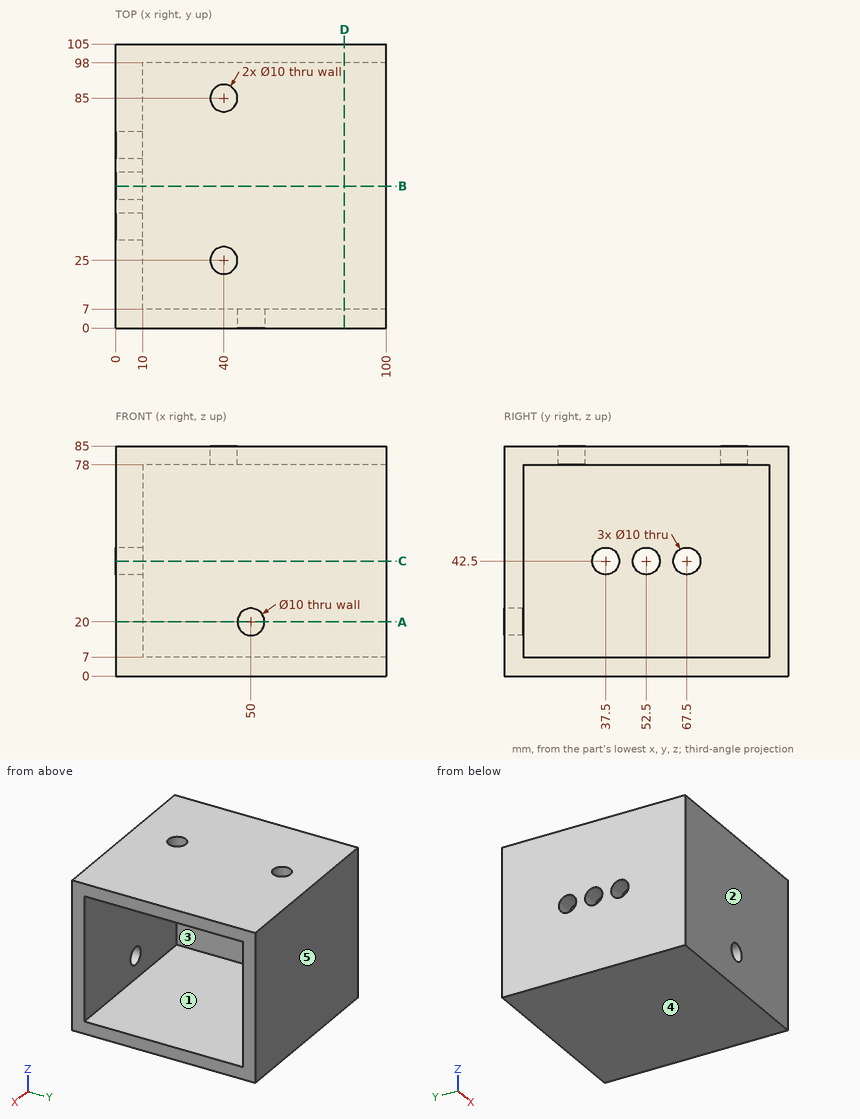
The figure shows three views and two pictorial views of one solid part (mm, origin at its lowest corner). Answer the questions. A direction names the side the tool comes from. Round coordinates to 2 decimals unless told otherwise and drop trailing zeros. Write each loop counter-clockwise with the first axis right and the second up, starting at its lowest first coordinate (ties: lowest second). Pieces come first, ordered by that corner, then holes. Notation, with made-up numbers: (30.25, -19.5) - (62.25, -19.5) arc R16 ccw to (62.25, 2.5) - close; hole circle Ø6 at (31, 55). An arc over 180 degrees is marked (long way). Use one line per item in the form item = value. Start each with the question number.
Item 1: A cutting plane is placed at A-A (z = 20). Write down the section's boundary in (x, y).
Item 2: Determine the mould class of the marked faces 3, 4 and 5 for opening direction Y: +Y half, -Y half, draft (parallel to the pull), parting line (faces both ways), or undercut.
Item 3: A cutting plane is placed at C-C (z = 42.5). Write down the section's boundary in (x, y), plus the area to 3 significant figures.
Item 4: Flat-ended cylindrical pins translate along their axes: pin 1 Ø4 at (y, z) = (28.5, 63) entering from +X; pin 2 Ø10 at (x, y) = (47.5, 73) entering from -Z; pin 3 Ø8 at (x, y) = (40, 25) entering from +Z. Find the tip coordinate at first contact, or state that the pin passes through.
Item 5: Find the intervals of material crossed by line 1 (Y direction, x = 40, z = 81.25); line 2 (Y direction, x = 5, z = 42); line 3 (Y direction, x = 87, z = 27), in increasing order. Write a range as [from, to].
Item 6: A cutting plane is placed at D-D (x = 84.5). Write down the section's boundary in (y, z), plus the area to 3 significant figures.
Item 7: A cutting plane is placed at B-B (y = 52.5). Write down the section's boundary in (x, z), plus the area to 3 significant figures.
Item 8: A tool of negligible diameter and unlimited length cuts with its end or side. For the marked faces 1 and 2, from which of +Z, -Z, +X, -X, +Y, -Y can it reach the whole face along a straight path? Write none if from no direction.
The answers:
q1.outline = (0, 0) - (45, 0) - (45, 7) - (10, 7) - (10, 98) - (100, 98) - (100, 105) - (0, 105) - close; (55, 0) - (100, 0) - (100, 7) - (55, 7) - close
q2.face_3 = undercut
q2.face_4 = draft
q2.face_5 = +Y half
q3.outline = (0, 0) - (100, 0) - (100, 7) - (10, 7) - (10, 32.5) - (0, 32.5) - close; (0, 42.5) - (10, 42.5) - (10, 47.5) - (0, 47.5) - close; (0, 57.5) - (10, 57.5) - (10, 62.5) - (0, 62.5) - close; (0, 72.5) - (10, 72.5) - (10, 98) - (100, 98) - (100, 105) - (0, 105) - close
q3.area = 2,010 mm^2
q4.pin_1 = 10
q4.pin_2 = 0
q4.pin_3 = 7
q5.line_1 = [0, 20], [30, 80], [90, 105]
q5.line_2 = [0, 32.53], [42.47, 47.53], [57.47, 62.53], [72.47, 105]
q5.line_3 = [0, 7], [98, 105]
q6.outline = (0, 0) - (105, 0) - (105, 85) - (0, 85) - close; hole (7, 7) - (98, 7) - (98, 78) - (7, 78) - close
q6.area = 2,460 mm^2
q7.outline = (0, 0) - (100, 0) - (100, 7) - (10, 7) - (10, 37.5) - (0, 37.5) - close; (0, 47.5) - (10, 47.5) - (10, 78) - (100, 78) - (100, 85) - (0, 85) - close
q7.area = 2,010 mm^2
q8.face_1 = +X
q8.face_2 = +Z, -Z, +X, -X, -Y
